Input: part model. Units: mm. Frame: model coordinates. Coordinates: 2 decimals unless noted, no trailing zeros. Loops run counter-clockwise (first coordinate to the right, second up) from the corner with the lowest first, then second, coordinate; pieces in that order, holes last. Notation, with made-up numbers: M 45.5,-12 L 83.5,-12 A24 cw 83.5,9 Z; hole C 86.5,-8.5 d2. An arc over 180 degrees is marked long. Use a Markdown table: item, result. Add a question column.
1. Section C-C on y = 7. Output: boundary loops of the cut face in (x, z).
2. Pin query (flat end, axial travel): pin 1 (3 mm diameter, centred on x = 2, z = 13, fed in from -Y); pin 2 (2 mm diameter, centred on x = 2.5, z = -11.5, fed in from -Y); pin 3 (2 mm diameter, centred on x = 2, y = 12.5, fed in from +Z). Return the tip coordinate at first contact, or that it passes through.
3. Section A-A on z = 0. Output: boundary loops of the cut face in (x, y) (3 decimals).
4. Section B-B on x = 5.75. State how many separate pieces and enclosed holes the cut face has, then the cut area to 3 significant figures.
5. Draft query along Z for faces 1 (the cylindrical face through (3.13, 7.38, -29.28)), 2 (the cylindrical face through (3.131, 12.655, 2.345)), 3 (the flat face through (3.131, -5.445, 18.624)). Return one class per face: +Z half, -Z half, draft (parallel to the pull), parting line (faces both ways), or undercut.
6. Line query: L1, parallel to Y at x = 5.75, z = -24; L2, parallel to Z at x = 5.25, y = 7; L3, parallel to Z at x = 3, y = 8. Output: solid intervals per line, ascending. Write a range as [from, to].
7. Section D-D on y = 14. Output: boundary loops of the cut face in (x, z).
Autodesk Inventor part; units mm, degrees
ref_plane "YZ Plane" through (0, 0, 0) normal (1, 0, 0) x (0, 1, 0)
ref_plane "XZ Plane" through (0, 0, 0) normal (0, 1, 0) x (-1, 0, 0)
ref_plane "XY Plane" through (0, 0, 0) normal (0, 0, 1) x (1, 0, 0)
sketch "Sketch1" plane through (0, 0, 0) normal (1, 0, 0) x (0, 1, 0)
  circle A0 centre (7.2644, 24.0085) radius 2.1082
  circle A1 centre (7.2644, -23.9975) radius 2.1082
  arc A2 (12.5476, 24.0085) -> (1.9812, 24.0085) centre (7.2644, 24.0085) ccw
  arc A3 (1.9812, -23.9975) -> (12.5476, -23.9975) centre (7.2644, -23.9975) ccw
  line L0 (12.5476, 24.0085) -> (19.008, 0.0055)
  line L1 (12.5476, -23.9975) -> (19.008, 0.0055)
  line L2 (1.9812, 24.0085) -> (-13.0815, 13.087)
  line L3 (-13.0815, -13.0759) -> (1.9812, -23.9975)
  arc A4 (-13.0815, 13.087) -> (-13.0815, -13.0759) centre (0, 0.0055) ccw
  circle A5 centre (7, 0) radius 6.1214
  point P0 (0, 0)
  dimension "d8" = 4.2164
  dimension "d11" = 4.2164
  dimension "d14" = 10.5664
  dimension "d15" = 10.5664
  dimension "d43" = 12.2428
extrude "Extrusion1" add sketch "Sketch1" along normal blind 6.35
fillet "Fillet1" radius 3.175 1 edges at (3.175, 19.008, 0.0055)
properties part number "MotorFixedPositionMount"
Answers below:
| question | item | result |
|---|---|---|
| 1 | outline | M 0,-29.27 L 6.35,-29.27 L 6.35,-26.09 L 0,-26.09 Z; M 0,-21.91 L 6.35,-21.91 L 6.35,-6.12 L 0,-6.12 Z; M 0,6.12 L 6.35,6.12 L 6.35,21.92 L 0,21.92 Z; M 0,26.1 L 6.35,26.1 L 6.35,29.29 L 0,29.29 Z |
| 2 | pin 1 | stops at y = -14.5 |
| 2 | pin 2 | stops at y = -15.23 |
| 2 | pin 3 | stops at z = 27.17 |
| 3 | outline | M 0,-18.5 L 6.35,-18.5 L 6.35,0.879 L 0,0.879 Z; M 0,13.121 L 6.35,13.121 L 6.35,18.895 L 0,18.895 Z |
| 4 | separate pieces | 1 |
| 4 | enclosed holes | 3 |
| 4 | area | 1,260 mm² |
| 5 | face 1 | -Z half |
| 5 | face 2 | undercut |
| 5 | face 3 | +Z half |
| 6 | L1 | y = [1.98, 5.16], [9.37, 12.55] |
| 6 | L2 | z = [-29.27, -26.09], [-21.91, -6.12], [6.12, 21.92], [26.1, 29.29] |
| 6 | L3 | z = [-29.23, -25.97], [-22.02, -6.04], [6.04, 22.03], [25.98, 29.24] |
| 7 | outline | M 0,-18.6 L 6.35,-18.6 L 6.35,18.61 L 0,18.61 Z |
